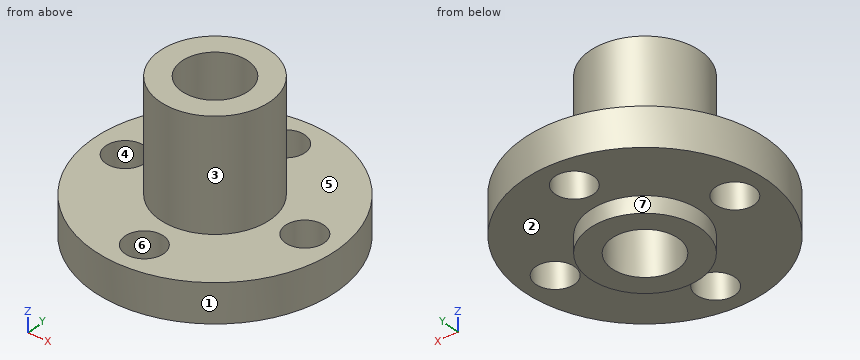
from build123d import *

# Parameters (mm, degrees)
F0_R     = 11
F0_R_2   = 4
F1_DEPTH = 3.5
F2_R     = 5
F2_R_2   = 3
F3_DEPTH = 10
F4_DEPTH = 5
F5_R     = 1.75
F6_DEPTH = 25


with BuildPart() as f1:
    # F0 (on Top) → F1 (new body)
    with BuildSketch(Plane.XY):
        Circle(F0_R)
        Circle(F0_R_2, mode=Mode.SUBTRACT)
    extrude(amount=F1_DEPTH)

    # F2 (on face) → F3 (join)
    with BuildSketch(Plane.XY.offset(3.5)):
        Circle(F2_R)
        Circle(F2_R_2, mode=Mode.SUBTRACT)
    extrude(amount=F3_DEPTH)

    # F2 (on face) → F4 (join)
    with BuildSketch(Plane.XY.offset(3.5)):
        Circle(F2_R)
        Circle(F2_R_2, mode=Mode.SUBTRACT)
    extrude(amount=-F4_DEPTH)

    # F5 (on face) → F6 (cut)
    with BuildSketch(Plane(origin=(0, 0, 0), x_dir=(1, 0, 0), z_dir=(0, 0, -1))):
        with Locations((-8, 0)):
            Circle(F5_R)
        with Locations((0, 8)):
            Circle(F5_R)
        with Locations((8, 0)):
            Circle(F5_R)
        with Locations((0, -8)):
            Circle(F5_R)
    extrude(amount=-F6_DEPTH, mode=Mode.SUBTRACT)


solid = f1.part
Check sheet for the modelled part. Datum: model origin and axes. Units: mm. Face numbers are marked on the shaded views. A direction names the side the tool comes from. Round coordinates to 2 decimals unless told otherwise and drop trailing zeros. Loops run counter-clockwise (first coordinate to the right, second up) from the corner with the lowest first, then second, coordinate; pieces in that order, holes last. Notation, with made-up numbers: M -18,71.5 L 0,71.5 A32 ccw 0,104.5 Z; hole C 67,-35 d10. An arc over 180 degrees is marked long. One line per question, with ' | ' between items. Start each with the question number.
Item 1: Scan lines: probe 1 along Y at (x, z) = (0, 0.85); probe 2 along Y at (x, z) = (0, 9.75); probe 3 along Z at (x, y) = (6.75, 1.75). Record each from-to range of solid material in increasing order.
Item 2: Section check C-C (z = 2). Record the boundary of the cut face in (x, y), and give its area (3 significant figures).
Item 3: Section check D-D (x = 7.25). Record the boundary of the cut face in (y, z), and give its area (3 significant figures).
Item 4: Gauge pin test, flat ends, axial feed: pin 1 Ø4 at (x, z) = (-5.5, 8.5) entering from -Y; pin 2 Ø2 at (x, y) = (-8.5, -2.5) entering from -Z; pin 3 Ø1.5 at (y, z) = (-2.5, 7.5) entering from +X; pin 4 Ø2 at (x, y) = (8, 0) entering from -Z. Record the tip position at first contact, or that the pin passes through.
Item 5: Release check for a two-part mould opening along X. For the marked faces 4, 5, 6 and 7 record: released by +X, released by -X, zero draft, split by the parting line, or undercut.
Item 6: Set-up check for the marked faces 1, 2 and 3: record each of +Z, -Z, +X, -X, +Y, -Y from which the full face is reachable in a straight line by a thin tool's end or side.
Item 7: Section check A-A (x = 0). Record the boundary of the cut face in (y, z).
Worked out:
1) probe 1: -11 to -9.75, -6.25 to -3, 3 to 6.25, 9.75 to 11 | probe 2: -5 to -3, 3 to 5 | probe 3: 0 to 3.5
2) outline: C 0,0 d22; hole C -8,0 d3.5; hole C 0,0 d6; hole C 0,-8 d3.5; hole C 0,8 d3.5; hole C 8,0 d3.5 | area: 313 mm^2
3) outline: M -8.27,0 L -1.58,0 L -1.58,3.5 L -8.27,3.5 Z; M 1.58,0 L 8.27,0 L 8.27,3.5 L 1.58,3.5 Z | area: 46.8 mm^2
4) pin 1: y = -3.57 | pin 2: z = 0 | pin 3: x = 4.68 | pin 4: through
5) face 4: undercut | face 5: zero draft | face 6: undercut | face 7: split by the parting line
6) face 1: +Z, -Z | face 2: -Z | face 3: +Z
7) outline: M -11,0 L -9.75,0 L -9.75,3.5 L -11,3.5 Z; M -6.25,0 L -5,0 L -5,-1.5 L -3,-1.5 L -3,13.5 L -5,13.5 L -5,3.5 L -6.25,3.5 Z; M 3,-1.5 L 5,-1.5 L 5,0 L 6.25,0 L 6.25,3.5 L 5,3.5 L 5,13.5 L 3,13.5 Z; M 9.75,0 L 11,0 L 11,3.5 L 9.75,3.5 Z
